from build123d import *

# Parameters (mm, degrees)
SKETCH1_W           = 923.925
SKETCH1_H           = 619.125
BOSS_EXTRUDE1_DEPTH = 3.175
SKETCH2_W           = 3.175
SKETCH2_H           = 619.125
BOSS_EXTRUDE2_DEPTH = 59.4
SKETCH3_W           = 917.575
SKETCH3_H           = 3.175
BOSS_EXTRUDE3_DEPTH = 59.4


with BuildPart() as part:
    # Sketch1 → Boss-Extrude1 (new body)
    with BuildSketch(Plane(origin=(0, 0, 0), x_dir=(1, 0, 0), z_dir=(0, 1, 0))):
        with Locations((461.9625, 309.5625)):
            Rectangle(SKETCH1_W, SKETCH1_H)
    extrude(amount=BOSS_EXTRUDE1_DEPTH)

    # Sketch2 → Boss-Extrude2 (add)
    with BuildSketch(Plane(origin=(0, 3.175, 0), x_dir=(1, 0, 0), z_dir=(0, 1, 0))):
        with Locations((1.5875, 309.5625)):
            Rectangle(SKETCH2_W, SKETCH2_H)
        with Locations((922.3375, 309.5625)):
            Rectangle(SKETCH2_W, SKETCH2_H)
    extrude(amount=BOSS_EXTRUDE2_DEPTH)

    # Sketch3 → Boss-Extrude3 (add)
    with BuildSketch(Plane(origin=(0, 3.175, 0), x_dir=(1, 0, 0), z_dir=(0, 1, 0))):
        with Locations((461.9625, 1.5875)):
            Rectangle(SKETCH3_W, SKETCH3_H)
        with Locations((461.9625, 617.5375)):
            Rectangle(SKETCH3_W, SKETCH3_H)
    extrude(amount=BOSS_EXTRUDE3_DEPTH)


solid = part.part
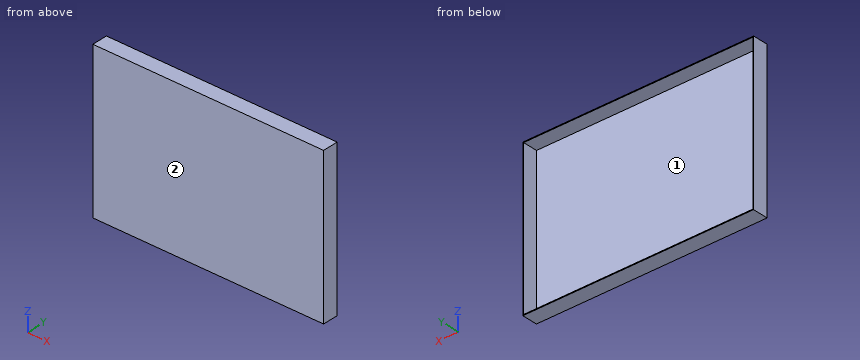
Source: CAD feature listing. Evaluate the final solid. Frame: model axes, mm. Face numbers are marked on the shaded views. Coordinates: 2 decimals unless noted, no trailing zeros. Order: outer loops, then holes, each group sorted by start corner. A loop starts at its lowest first (then second) coordinate and runs counter-clockwise, first axis right, second up. Notation, with made-up numbers: M -25.75,-7 L -17.75,-7 A19 cw -17.75,19 Z; hole C 39,45 d7. An arc over 180 degrees is marked long. Write each question's results on one line, items separated by ' | '. Start each with the question number.
1. Draft query along Z for the marked faces 1 and 2. Return one class per face: +Z half, -Z half, draft (parallel to the pull), parting line (faces both ways), or undercut.
2. Section B-B, the plane y = 13.5. Return the cut outline in (x, z) (3 decimals).
3. Section A-A, the plane z = -234.5. Return the cut outline in (x, y) (3 decimals).
4. Material intervals for L1, parallel to Z at x = 421, y = 12 (3 decimals); L2, parallel to X at y = 17, z = -269.5 (3 decimals); L3, parallel to Y at x = 110, z = -117 (3 decimals), sorted ascending.
5. Section C-C, the plane x = 82. Return the cut outline in (y, z) (3 decimals), then the cut area to 3 significant figures.
6. Pin query (flat end, axial travel): pin 1 (8 mm diameter, centred on x = 609.5, z = -136, fed in from +Y) (3 decimals). Return the tip coordinate at first contact, or that it passes through.
Solution:
1) face 1: undercut | face 2: draft
2) outline: M 0,-619.125 L 923.925,-619.125 L 923.925,0 L 0,0 Z; hole M 3.175,-615.95 L 920.75,-615.95 L 920.75,-3.175 L 3.175,-3.175 Z
3) outline: M 0,0 L 923.925,0 L 923.925,62.575 L 920.75,62.575 L 920.75,3.175 L 3.175,3.175 L 3.175,62.575 L 0,62.575 Z
4) L1: -619.125 to -615.95, -3.175 to 0 | L2: 0 to 3.175, 920.75 to 923.925 | L3: 0 to 3.175
5) outline: M 0,-619.125 L 62.575,-619.125 L 62.575,-615.95 L 3.175,-615.95 L 3.175,-3.175 L 62.575,-3.175 L 62.575,0 L 0,0 Z | area: 2,340 mm²
6) pin 1: y = 3.175
